```python
from build123d import *

# Parameters (mm, degrees)
SKETCH1_R           = 1.575
BOSS_EXTRUDE1_DEPTH = 6
CUT_EXTRUDE3_START  = -3
SKETCH2_R           = 2.9
SKETCH2_R_2         = 1.575
CUT_EXTRUDE3_DEPTH  = 3
CUT_EXTRUDE4_START  = -3
SKETCH2_3_R         = 2.9
SKETCH2_3_R_2       = 1.575
CUT_EXTRUDE4_DEPTH  = 3
SKETCH3_W           = 36.8
SKETCH3_H           = 4
BOSS_EXTRUDE2_DEPTH = 16
CUT_EXTRUDE5_DEPTH  = 10
FILLET2_R           = 1


with BuildPart() as part:
    # Sketch1 → Boss-Extrude1 (new body)
    # profile 1 of 2: a face of its own
    with BuildSketch(Plane.XY):
        with BuildLine():
            ThreePointArc((18.4, 0), (0, 18.4), (-18.4, 0))
            ThreePointArc((-18.4, 0), (0, -18.4), (18.4, 0))
        make_face()
        with Locations((-7.75, -13.423393759)):
            Circle(SKETCH1_R, mode=Mode.SUBTRACT)
        with Locations((7.75, -13.423393759)):
            Circle(SKETCH1_R, mode=Mode.SUBTRACT)
        with Locations((-15.5, 0)):
            Circle(SKETCH1_R, mode=Mode.SUBTRACT)
        with Locations((-7.75, 13.423393759)):
            Circle(SKETCH1_R, mode=Mode.SUBTRACT)
        with BuildLine():
            ThreePointArc((6.25, -7.1), (0, -13.35), (-6.25, -7.1))
            Line((-6.25, -7.1), (-6.25, 7.1))
            ThreePointArc((-6.25, 7.1), (0, 13.35), (6.25, 7.1))
            Line((6.25, 7.1), (6.25, -7.1))
        make_face(mode=Mode.SUBTRACT)
        with Locations((15.5, 0)):
            Circle(SKETCH1_R, mode=Mode.SUBTRACT)
        with Locations((7.75, 13.423393759)):
            Circle(SKETCH1_R, mode=Mode.SUBTRACT)
    # profile 2 of 2: a face of its own
    with BuildSketch(Plane.XY):
        with BuildLine():
            ThreePointArc((18.4, 0), (0, -18.4), (-18.4, 0))
            Line((-18.4, 0), (-18.4, -19))
            Line((-18.4, -19), (18.4, -19))
            Line((18.4, -19), (18.4, 0))
        make_face()
    extrude(amount=BOSS_EXTRUDE1_DEPTH)

    # Sketch2 → Cut-Extrude3 (cut)
    # profile 1 of 12: a face of its own
    with BuildSketch(Plane.XY.offset(6).offset(CUT_EXTRUDE3_START)):
        with Locations((-15.5, 0)):
            Circle(SKETCH2_R)
        with Locations((-15.5, 0)):
            Circle(SKETCH2_R_2, mode=Mode.SUBTRACT)
    # profile 2 of 12: a face of its own
    with BuildSketch(Plane.XY.offset(6).offset(CUT_EXTRUDE3_START)):
        with BuildLine():
            ThreePointArc((-18.4, 0), (-17.550609665, 2.050609665), (-15.5, 2.9))
            Line((-15.5, 2.9), (-18.17003027, 2.9))
            ThreePointArc((-18.17003027, 2.9), (-18.342417466, 1.454551999), (-18.4, 0))
        make_face()
    # profile 3 of 12: a face of its own
    with BuildSketch(Plane.XY.offset(6).offset(CUT_EXTRUDE3_START)):
        with BuildLine():
            ThreePointArc((-15.5, -2.9), (-17.550609665, -2.050609665), (-18.4, 0))
            Line((-18.4, 0), (-18.4, -2.9))
            Line((-18.4, -2.9), (-15.5, -2.9))
        make_face()
    # profile 4 of 12: a face of its own
    with BuildSketch(Plane.XY.offset(6).offset(CUT_EXTRUDE3_START)):
        with BuildLine():
            ThreePointArc((-6.573541464, 17.185707801), (-7.911529831, 16.612275453), (-9.200000154, 15.934867341))
            ThreePointArc((-9.200000154, 15.934867341), (-6.999424855, 16.224578678), (-5.238526329, 14.873393759))
            Line((-5.238526329, 14.873393759), (-6.573541464, 17.185707801))
        make_face()
    # profile 5 of 12: a face of its own
    with BuildSketch(Plane.XY.offset(6).offset(CUT_EXTRUDE3_START)):
        with BuildLine():
            ThreePointArc((-9.200000154, 15.934867341), (-10.430887789, 15.157723442), (-11.596488806, 14.285707801))
            Line((-11.596488806, 14.285707801), (-10.261473671, 11.973393759))
            ThreePointArc((-10.261473671, 11.973393759), (-10.551184919, 14.173968903), (-9.200000154, 15.934867341))
        make_face()
    # profile 6 of 12: a face of its own
    with BuildSketch(Plane.XY.offset(6).offset(CUT_EXTRUDE3_START)):
        with Locations((-7.75, 13.423393759)):
            Circle(SKETCH2_R)
        with Locations((-7.75, 13.423393759)):
            Circle(SKETCH2_R_2, mode=Mode.SUBTRACT)
    # profile 7 of 12: a face of its own
    with BuildSketch(Plane.XY.offset(6).offset(CUT_EXTRUDE3_START)):
        with BuildLine():
            ThreePointArc((9.200000155, 15.93486734), (7.911529831, 16.612275453), (6.573541464, 17.185707801))
            Line((6.573541464, 17.185707801), (5.238526329, 14.873393759))
            ThreePointArc((5.238526329, 14.873393759), (6.999424856, 16.224578678), (9.200000155, 15.93486734))
        make_face()
    # profile 8 of 12: a face of its own
    with BuildSketch(Plane.XY.offset(6).offset(CUT_EXTRUDE3_START)):
        with Locations((7.75, 13.423393759)):
            Circle(SKETCH2_R)
        with Locations((7.75, 13.423393759)):
            Circle(SKETCH2_R_2, mode=Mode.SUBTRACT)
    # profile 9 of 12: a face of its own
    with BuildSketch(Plane.XY.offset(6).offset(CUT_EXTRUDE3_START)):
        with BuildLine():
            ThreePointArc((11.596488806, 14.285707801), (10.430887789, 15.157723441), (9.200000155, 15.93486734))
            ThreePointArc((9.200000155, 15.93486734), (10.261473716, 14.873393681), (10.65, 13.423393759))
            ThreePointArc((10.65, 13.423393759), (10.551184896, 12.672818528), (10.261473671, 11.973393759))
            Line((10.261473671, 11.973393759), (11.596488806, 14.285707801))
        make_face()
    # profile 10 of 12: a face of its own
    with BuildSketch(Plane.XY.offset(6).offset(CUT_EXTRUDE3_START)):
        with BuildLine():
            ThreePointArc((18.4, 0), (18.342417466, 1.454551999), (18.17003027, 2.9))
            Line((18.17003027, 2.9), (15.5, 2.9))
            ThreePointArc((15.5, 2.9), (17.550609665, 2.050609665), (18.4, 0))
        make_face()
    # profile 11 of 12: a face of its own
    with BuildSketch(Plane.XY.offset(6).offset(CUT_EXTRUDE3_START)):
        with Locations((15.5, 0)):
            Circle(SKETCH2_R)
        with Locations((15.5, 0)):
            Circle(SKETCH2_R_2, mode=Mode.SUBTRACT)
    # profile 12 of 12: a face of its own
    with BuildSketch(Plane.XY.offset(6).offset(CUT_EXTRUDE3_START)):
        with BuildLine():
            Line((18.4, -2.9), (18.4, 0))
            ThreePointArc((18.4, 0), (17.550609665, -2.050609665), (15.5, -2.9))
            Line((15.5, -2.9), (18.4, -2.9))
        make_face()
    extrude(amount=CUT_EXTRUDE3_DEPTH, mode=Mode.SUBTRACT)

    # Sketch2<3> → Cut-Extrude4 (cut)
    # profile 1 of 2: a face of its own
    with BuildSketch(Plane.XY.offset(6).offset(CUT_EXTRUDE4_START)):
        with Locations((7.75, -13.423393759)):
            Circle(SKETCH2_3_R)
        with Locations((7.75, -13.423393759)):
            Circle(SKETCH2_3_R_2, mode=Mode.SUBTRACT)
    # profile 2 of 2: a face of its own
    with BuildSketch(Plane.XY.offset(6).offset(CUT_EXTRUDE4_START)):
        with Locations((-7.75, -13.423393759)):
            Circle(SKETCH2_3_R)
    extrude(amount=CUT_EXTRUDE4_DEPTH, mode=Mode.SUBTRACT)

    # Sketch3 → Boss-Extrude2 (add)
    with BuildSketch(Plane.XY):
        with Locations((0, -18.423393759)):
            Rectangle(SKETCH3_W, SKETCH3_H)
    extrude(amount=BOSS_EXTRUDE2_DEPTH)

    # Sketch4 → Cut-Extrude5 (cut)
    with BuildSketch(Plane(origin=(0, -16.423393759, 0), x_dir=(1, 0, 0), z_dir=(0, 1, 0))):
        with BuildLine():
            Line((-4.45, -8.5), (-4.45, -13.5))
            ThreePointArc((-4.45, -13.5), (-6, -15.05), (-7.55, -13.5))
            Line((-7.55, -13.5), (-7.55, -8.5))
            ThreePointArc((-7.55, -8.5), (-6, -6.95), (-4.45, -8.5))
        make_face()
        with BuildLine():
            Line((4.45, -8.5), (4.45, -13.5))
            ThreePointArc((4.45, -13.5), (6, -15.05), (7.55, -13.5))
            Line((7.55, -13.5), (7.55, -8.5))
            ThreePointArc((7.55, -8.5), (6, -6.95), (4.45, -8.5))
        make_face()
    extrude(amount=-CUT_EXTRUDE5_DEPTH, mode=Mode.SUBTRACT)

    # Fillet2
    fillet2_edges = [part.edges().sort_by_distance(p)[0] for p in [
        (-18.4, -2.9, 4.5),
        (-18.17003027, 2.9, 4.5),
        (-11.596488806, 14.285707801, 4.5),
        (-6.573541464, 17.185707801, 4.5),
        (6.573541464, 17.185707801, 4.5),
        (11.596488806, 14.285707801, 4.5),
        (18.17003027, 2.9, 4.5),
        (18.4, -2.9, 4.5),
    ]]
    fillet(fillet2_edges, radius=FILLET2_R)


solid = part.part
```
Check sheet for the modelled part. Datum: model origin and axes. Units: mm. A direction names the side the tool comes from. Give positions to 0.01 mm unless a question says otherwise; leave off trailing zeros. Write each loop counter-clockwise with the first axis right and the second up, starting at its lowest first coordinate (ties: lowest second). Pieces come first, ordered by that corner, then holes. Notation, with made-up numbers: (-22.75, 89.25) -> (29.25, 89.25) arc R11 cw to (29.25, 109.25) -> close; hole circle Ø11 at (25.5, 3). An arc over 180 degrees is marked (long way). Use CSV: the item, a comma, the result in double quotes. Start each with the question number.
Q1. Release check for a two-part mould opening along Z. For faces 6 (the flat face through (17, 1, 3)), 7 (the cylindrical face through (-14.045, -0.603, 1.479)), 8 (the cylindrical face through (5.97, -18.4, 15.05)) record: +Z half, -Z half, draft (parallel to the pull), parting line (faces both ways), or undercut.
Q2. Scan lines: line 1 along Y through (x, z) = (-7.75, 2.45); line 2 along X through (y, z) = (11, 5.25); line 3 along Y through (x, z) = (-9, 1). Record each from-to range of solid material in increasing order.
Q3. Cross-section at A-A on y = -5. Enter the section's corners in (x, z).
Q4. Tool access check on faces 1 (the cylindrical face through (-9.887, -11.463, 4.479)), 2 (the flat face through (-10.63, 12.61, 4.48)), 3 (the cylindrical face through (-0.14, 13.35, 2.96)), 4 (the cylindrical face through (6.03, -18.4, 6.95)), 5 (the flat face through (16, 2.9, 4)). Record the directions out of +Z, -Z, +X, -X, +Y, -Y that give a thin tool (end or side, any length) a straight path to the whole face; none if there is none.
Q5. Cross-section at D-D on x = 16.5. Enter the section's corners in (y, z).
Q6. Cross-section at B-B on x = 2. Enter the section's corners in (y, z).
Q7. Depth check by flat-ended pin: P1, Ø17.5, axis at x = -2, y = -2.5, coming from the +Z side; P2, Ø5, axis at x = -7.75, y = 13.42, coming from the -Z side; P3, Ø1.5, axis at x = 16.5, z = 4.5, coming from the +Y side; P4, Ø8, axis at x = 2.5, z = 12, coming from the +Y side. Enter the tip coordinate at first touch or a pass-through.
Q8. Cross-section at C-C on z = 1.75. Enter the section's corners in (x, y) (3 decimals), and give its area (3 significant figures).
Working result:
1,face 6,"+Z half"
1,face 7,"draft"
1,face 8,"undercut"
2,line 1,"y = -20.42 to -15, -11.85 to 11.85, 15 to 16.69"
2,line 2,"x = -14.75 to -9.34, -6.16 to -4.88, 4.88 to 6.16, 9.34 to 14.75"
2,line 3,"y = -20.42 to -14.38, -12.47 to 12.47, 14.38 to 16.05"
3,outline,"(-18.4, 0) -> (-6.25, 0) -> (-6.25, 6) -> (-18.4, 6) -> close; (6.25, 0) -> (18.4, 0) -> (18.4, 6) -> (6.25, 6) -> close"
4,face 1,"+Z"
4,face 2,"+Z, +Y"
4,face 3,"+Z, -Z"
4,face 4,"+Y, -Y"
4,face 5,"+Z, +X"
5,outline,"(-20.42, 0) -> (-1.22, 0) -> (-1.22, 3) -> (-2.9, 3) -> (-2.9, 6) -> (-16.42, 6) -> (-16.42, 16) -> (-20.42, 16) -> close; (1.22, 0) -> (8.14, 0) -> (8.14, 6) -> (2.9, 6) -> (2.9, 3) -> (1.22, 3) -> close"
6,outline,"(-20.42, 0) -> (-13.02, 0) -> (-13.02, 6) -> (-16.42, 6) -> (-16.42, 16) -> (-20.42, 16) -> close; (13.02, 0) -> (18.29, 0) -> (18.29, 6) -> (13.02, 6) -> close"
7,P1,"stops at z = 6"
7,P2,"stops at z = 0"
7,P3,"stops at y = 9.51"
7,P4,"stops at y = -16.42"
8,outline,"(-18.4, -20.423) -> (18.4, -20.423) -> (18.4, 0) arc R18.4 ccw to (-18.4, 0) -> close; hole circle Ø3.15 at (-15.5, 0); hole circle Ø3.15 at (-7.75, -13.423); hole circle Ø3.15 at (-7.75, 13.423); hole (-6.25, -7.1) arc R6.25 ccw to (6.25, -7.1) -> (6.25, 7.1) arc R6.25 ccw to (-6.25, 7.1) -> close; hole circle Ø3.15 at (7.75, -13.423); hole circle Ø3.15 at (7.75, 13.423); hole circle Ø3.15 at (15.5, 0)"
8,area,"936 mm^2"
